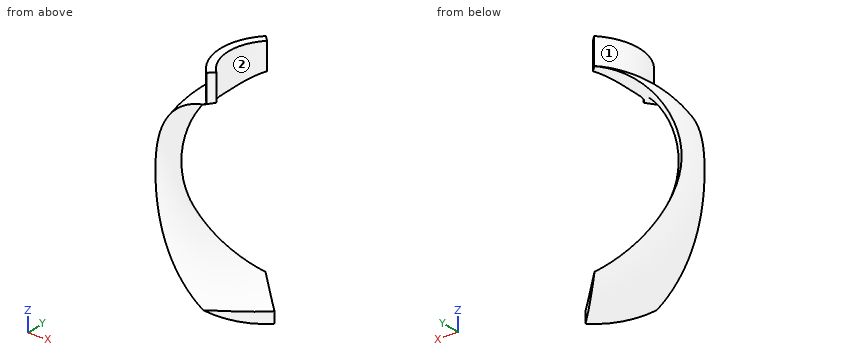
```python
from build123d import *

# Parameters (mm, degrees)
F1_ANGLE_BACK = 45
F1_ANGLE      = 90
F2_ANGLE_BACK = 90
F2_ANGLE      = 180
F4_DEPTH      = 25


with BuildPart() as f1:
    # F0 (on Front) → F1 (revolve)
    with BuildSketch(Plane.XZ, mode=Mode.PRIVATE) as f1_sk:
        with BuildLine():
            Line((50, 42.9009879801), (50, 53.4044873264))
            Line((50, 53.4044873264), (26, 53.4044873264))
            Line((26, 53.4044873264), (26, 41.4702073618))
            ThreePointArc((26, 41.4702073618), (3.6355603381, -12.5223261848), (50, -48.0990120199))
            Line((50, -48.0990120199), (50, -43.0990120199))
            ThreePointArc((50, -43.0990120199), (7, -0.0990120199), (50, 42.9009879801))
        make_face()
    revolve(f1_sk.sketch.rotate(Axis((50, 0, -0.0990120199), (0, 0, -1)), -F1_ANGLE_BACK), axis=Axis((50, 0, -0.0990120199), (0, 0, -1)), revolution_arc=F1_ANGLE)

    # F0 (on Front) → F2 (revolve, cut)
    with BuildSketch(Plane.XZ, mode=Mode.PRIVATE) as f2_sk:
        with BuildLine():
            Line((50, -43.0990120199), (50, 42.9009879801))
            ThreePointArc((50, 42.9009879801), (7, -0.0990120199), (50, -43.0990120199))
        make_face()
    revolve(f2_sk.sketch.rotate(Axis((0, 0, -0.0990120199), (0, 0, -1)), -F2_ANGLE_BACK), axis=Axis((0, 0, -0.0990120199), (0, 0, -1)), revolution_arc=F2_ANGLE, mode=Mode.SUBTRACT)

    # F3 (on face) → F4 (cut)
    with BuildSketch(Plane.XY.offset(53.4044873264)):
        with BuildLine():
            Line((50, 0), (35.5043109857, 14.4956890143))
            ThreePointArc((35.5043109857, 14.4956890143), (29.5, 0), (35.5043109857, -14.4956890143))
            Line((35.5043109857, -14.4956890143), (50, 0))
        make_face()
    extrude(amount=-F4_DEPTH, mode=Mode.SUBTRACT)


solid = f1.part
```
CAD build for the part. Positions are in the model's coordinates, mm. Face numbers are marked on the shaded views. A direction names the side the tool comes from. Coordinates: 2 decimals unless noted, no trailing zeros. Write each loop counter-clockwise with the first axis right and the second up, starting at its lowest first coordinate (ties: lowest second). Pieces come first, ordered by that corner, then holes. Notation, with made-up numbers: (16.5, 42) -> (23.5, 42) arc R16 cw to (23.5, 66) -> close; hole circle Ø5 at (48.25, 2.5). An arc over 180 degrees is marked (long way). Return JSON: item names as keys, results as strings. Group by question number.
Q1. Drill centre lines: line 1 (Z direction, x = 30.5, y = -10.5); line 2 (Z direction, x = 12.5, y = -6); line 3 (X direction, y = -1, z = 48.5). Where is each one in solid material? Low to high.
Q2. Which spindle directions (+Z, -Z, +X, -X, +Y, -Y) get a long thin tool onto all of the face, cutting with end or side? Do the marked faces 1 and 2. Say none if no direction does.
Q3. Cut at C-C, the plane z = -30. Give the cut face in (x, y).
Q4. Flat gauge pins, fed straight in: pin 1 (3 mm diameter, centred on x = 42.5, y = -2, fed in from -Z); pin 2 (5 mm diameter, centred on x = 43.5, y = 13.5, fed in from +Z); pin 3 (3 mm diameter, centred on y = 1, z = 7.5, fed in from +X); pin 4 (10 mm diameter, centred on x = 11, z = -4, fed in from +Y). Where does each tip first touch, or does it go through?
Q5. Cut at A-A, the plane z = 47. Give the cut face in (x, y).
Returned:
{
 "1": {"line 1": "z = -42.68 to -39.27, 39.07 to 53.4", "line 2": "z = -29.45 to -23.41, 23.21 to 29.26", "line 3": "x = 26.02 to 29.52"},
 "2": {"face 1": "+Z, -X", "face 2": "+Z, +X"},
 "3": {"outline": "(14.55, -12.37) arc R19.1 ccw to (14.55, 12.37) arc R37.55 ccw to start"},
 "4": {"pin 1": "stops at z = -47.69", "pin 2": "passes through", "pin 3": "stops at x = 7.94", "pin 4": "stops at y = 3.99"},
 "5": {"outline": "(33.03, -16.97) -> (35.5, -14.5) arc R20.5 cw to (35.5, 14.5) -> (33.03, 16.97) arc R24 ccw to start"}
}
